Geometry check sheet. Reference: the model listing, model coordinates, mm. Face numbers are marked on the shaded views. A direction names the side the tool comes from. Round coordinates to 2 decimals unless told otherwise and drop trailing zeros. Loops run counter-clockwise (first coordinate to the right, second up) from the corner with the lowest first, then second, coordinate; pieces in that order, holes last.
```python
from build123d import *

# Parameters (mm, degrees)
SKETCH_1_R          = 165
EXTRUDE_1_DEPTH     = 16.6
SKETCH_2_R          = 30
CUT_EXTRUDE_1_DEPTH = 6.6
SKETCH_3_R          = 2.5
SKETCH_3_R_2        = 2
CUT_EXTRUDE_2_DEPTH = 234.559414283
SKETCH_4_W          = 107
SKETCH_4_H          = 97.5
EXTRUDE_2_DEPTH     = 34.3
SKETCH_5_W          = 98
SKETCH_5_H          = 92.5
CUT_EXTRUDE_3_DEPTH = 27.7
SKETCH_6_R          = 29.5
CUT_EXTRUDE_4_DEPTH = 6.6
FILLET_1_R          = 10


with BuildPart() as part:
    # 草图1 → 凸台-拉伸1 (new body)
    with BuildSketch(Plane(origin=(0, 0, 0), x_dir=(1, 0, 0), z_dir=(0, 1, 0))):
        with Locations(Location((0, 0, 0), (0, 0, 90))):
            Circle(SKETCH_1_R)
    extrude(amount=EXTRUDE_1_DEPTH)

    # 草图2 → 切除-拉伸1 (cut)
    with BuildSketch(Plane.XZ):
        with Locations(Location((0, 0, 0), (0, 0, 270))):
            Circle(SKETCH_2_R)
    extrude(amount=-CUT_EXTRUDE_1_DEPTH, mode=Mode.SUBTRACT)

    # 草图3 → 切除-拉伸2 (cut, through all)
    with BuildSketch(Plane.XZ.offset(-6.6)):
        with Locations(Location((0, 0, 0), (0, 0, 270))):
            Circle(SKETCH_3_R)
        with Locations(Location((0, 17.25, 0), (0, 0, 270))):
            Circle(SKETCH_3_R_2)
        with Locations(Location((0, -17.25, 0), (0, 0, 270))):
            Circle(SKETCH_3_R_2)
    extrude(amount=-CUT_EXTRUDE_2_DEPTH, mode=Mode.SUBTRACT)

    # 草图4 → 凸台-拉伸2 (add)
    with BuildSketch(Plane(origin=(10, 0, 0), x_dir=(0, 0, -1), z_dir=(1, 0, 0))):
        with Locations((0, 65.35)):
            Rectangle(SKETCH_4_W, SKETCH_4_H)
    extrude(amount=EXTRUDE_2_DEPTH)

    # 草图5 → 切除-拉伸3 (cut)
    with BuildSketch(Plane(origin=(44.3, 0, 0), x_dir=(0, 0, -1), z_dir=(1, 0, 0))):
        with Locations((0, 62.85)):
            Rectangle(SKETCH_5_W, SKETCH_5_H)
    extrude(amount=-CUT_EXTRUDE_3_DEPTH, mode=Mode.SUBTRACT)

    # 草图6 → 切除-拉伸4 (cut)
    with BuildSketch(Plane(origin=(16.6, 0, 0), x_dir=(0, 0, -1), z_dir=(1, 0, 0))):
        with Locations((0, 62.85)):
            Circle(SKETCH_6_R)
    extrude(amount=-CUT_EXTRUDE_4_DEPTH, mode=Mode.SUBTRACT)

    # 圆角1
    fillet_1_edges = [part.edges().sort_by_distance(p)[0] for p in [
        (27.15, 114.1, 53.5),
        (27.15, 114.1, -53.5),
    ]]
    fillet(fillet_1_edges, radius=FILLET_1_R)


solid = part.part
```
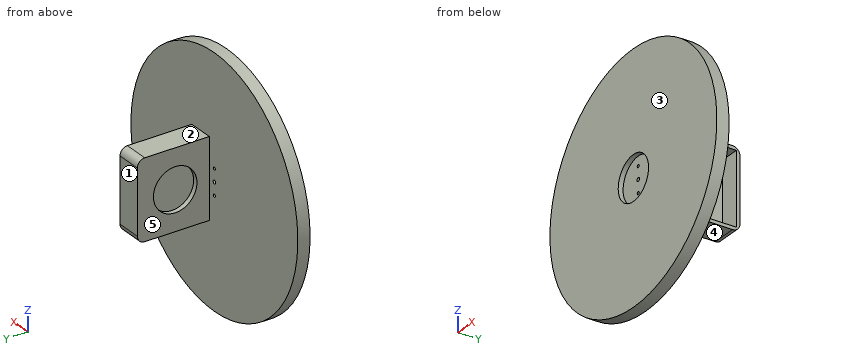
1) Access from +Z, -Z, +X, -X, +Y, -Y to the whole of each face (thin tool, end or side, straight path). Record for the marked faces 1, 2, 3, 4 and 5.
Report:
face 1: +Z, -Z, +X, -X, +Y
face 2: +Z, +X, -X, +Y
face 3: +Z, -Z, +X, -X, -Y
face 4: -Z, +X, -X, +Y
face 5: +Z, -Z, -X, +Y
2) Sectioned sample at A-A, the plane y = 62.85. Record the cut outline in (x, z).
Report:
outline: (10, -53.5) - (44.3, -53.5) - (44.3, -49) - (16.6, -49) - (16.6, -29.5) - (10, -29.5) - close; (10, 29.5) - (16.6, 29.5) - (16.6, 49) - (44.3, 49) - (44.3, 53.5) - (10, 53.5) - close
3) Gauge pin test, flat ends, axial feed: pin 1 (10.5 mm diameter, centred on x = 27.5, y = 75.5, fed in from +Z); pin 2 (10 mm diameter, centred on y = 52.5, z = -37.5, fed in from -X); pin 3 (10 mm diameter, centred on x = -31.5, z = 128, fed in from +Y); pin 4 (2.5 mm diameter, centred on x = 0, z = 17.25, fed in from +Y). Record the tip position at first contact, or that the pin passes through.
Report:
pin 1: stops at z = 53.5
pin 2: stops at x = 10
pin 3: stops at y = 16.6
pin 4: passes through
4) Sectioned sample at D-D, the plane y = 84.5. Record the cut outline in (x, z).
Report:
outline: (10, -53.5) - (44.3, -53.5) - (44.3, -49) - (16.6, -49) - (16.6, -20.04) - (10, -20.04) - close; (10, 20.04) - (16.6, 20.04) - (16.6, 49) - (44.3, 49) - (44.3, 53.5) - (10, 53.5) - close
5) Sectioned sample at C-C, the plane z = 35. Record the cut outline in (x, y).
Report:
outline: (-161.25, 0) - (161.25, 0) - (161.25, 16.6) - (16.6, 16.6) - (16.6, 109.1) - (44.3, 109.1) - (44.3, 114.1) - (10, 114.1) - (10, 16.6) - (-161.25, 16.6) - close
6) Sectioned sample at B-B, the plane y = 20.5. Record the cut outline in (x, z), then the cut area to 4 significant figures.
Report:
outline: (10, -53.5) - (44.3, -53.5) - (44.3, -49) - (16.6, -49) - (16.6, 49) - (44.3, 49) - (44.3, 53.5) - (10, 53.5) - close
area: 955.5 mm2
7) Scan lines: line 1 along Y through (x, z) = (11.5, 0); line 2 along Y through (x, z) = (20.5, 21); line 3 along X through (y, z) = (11, 0). Record each from-to range of solid material in increasing order.
Report:
line 1: y = 6.6 to 33.35, 92.35 to 114.1
line 2: y = 6.6 to 16.6, 109.1 to 114.1
line 3: x = -165 to -2.5, 2.5 to 165
